```python
from build123d import *

# Parameters (mm, degrees)
SKETCH_2_OUTSIDE_W   = 46.494
SKETCH_2_OUTSIDE_H   = 46.494
SKETCH_2_OUTSIDE_W_2 = 10
SKETCH_2_OUTSIDE_H_2 = 5
CUT_EXTRUDE_1_DEPTH  = 10
SKETCH_3_OUTSIDE_W   = 46.494
SKETCH_3_OUTSIDE_H   = 46.494
SKETCH_3_OUTSIDE_W_2 = 5
SKETCH_3_OUTSIDE_H_2 = 20
CUT_EXTRUDE_2_DEPTH  = 8.5
CUT_EXTRUDE_3_DEPTH  = 131.817621137


with BuildPart() as part:
    # Эскиз1 → Повернуть2 (revolve)
    with BuildSketch(Plane.XY, mode=Mode.PRIVATE) as revolve_2_sk:
        with BuildLine():
            Line((-3.5, 8.570714214), (-3.5, 23.570714214))
            Line((-3.5, 23.570714214), (-9, 23.570714214))
            Line((-9, 23.570714214), (-9, 25.570714214))
            Line((-9, 25.570714214), (-1.5, 25.570714214))
            Line((-1.5, 25.570714214), (-1.5, 71.070714214))
            Line((-1.5, 71.070714214), (-6, 71.070714214))
            Line((-6, 71.070714214), (-6, 105.570714214))
            Line((-6, 105.570714214), (-9, 105.570714214))
            Line((-9, 105.570714214), (-9, 108.570714214))
            Line((-9, 108.570714214), (-8, 108.570714214))
            Line((-8, 108.570714214), (-8, 123.570714214))
            Line((-8, 123.570714214), (-4.791361199, 123.570714214))
            ThreePointArc((-4.791361199, 123.570714214), (-4.009141362, 127.987772671), (0, 130))
            Line((0, 130), (0, 125))
            Line((0, 125), (0, 0))
            ThreePointArc((0, 0), (-4.628907596, 3.109705191), (-3.5, 8.570714214))
        make_face()
    revolve(revolve_2_sk.sketch.rotate(Axis((0, 125, 0), (0, -1, 0)), 270), axis=Axis((0, 125, 0), (0, -1, 0)))

    # Эскиз2 outside → Вырез-Вытянуть1 (cut)
    with BuildSketch(Plane(origin=(0, 123.570714214, 0), x_dir=(1, 0, 0), z_dir=(0, 1, 0))):
        Rectangle(SKETCH_2_OUTSIDE_W, SKETCH_2_OUTSIDE_H)
        Rectangle(SKETCH_2_OUTSIDE_W_2, SKETCH_2_OUTSIDE_H_2, mode=Mode.SUBTRACT)
    extrude(amount=CUT_EXTRUDE_1_DEPTH, mode=Mode.SUBTRACT)

    # Эскиз3 outside → Вырез-Вытянуть2 (cut)
    with BuildSketch(Plane(origin=(0, 0, 0), x_dir=(1, 0, 0), z_dir=(0, 1, 0))):
        Rectangle(SKETCH_3_OUTSIDE_W, SKETCH_3_OUTSIDE_H)
        Rectangle(SKETCH_3_OUTSIDE_W_2, SKETCH_3_OUTSIDE_H_2, mode=Mode.SUBTRACT)
    extrude(amount=CUT_EXTRUDE_2_DEPTH, mode=Mode.SUBTRACT)

    # Эскиз4 → Вырез-Вытянуть3 (cut, through all)
    with BuildSketch(Plane(origin=(2.5, 0, 0), x_dir=(0, 0, -1), z_dir=(1, 0, 0))):
        with BuildLine():
            Line((-1.198957881, 7.334936491), (1.198957881, 7.334936491))
            ThreePointArc((1.198957881, 7.334936491), (3, 4.584936491), (1.198957881, 1.834936491))
            Line((1.198957881, 1.834936491), (-1.198957881, 1.834936491))
            ThreePointArc((-1.198957881, 1.834936491), (-3, 4.584936491), (-1.198957881, 7.334936491))
        make_face()
    extrude(amount=-CUT_EXTRUDE_3_DEPTH, mode=Mode.SUBTRACT)


solid = part.part
```
Input: part model. Units: mm. Frame: model coordinates. A direction names the side the tool comes from. Give positions to 0.01 mm unless a question says otherwise; leave off trailing zeros. Loops run counter-clockwise (first coordinate to the right, second up) from the corner with the lowest first, then second, coordinate; pieces in that order, holes last. Notation, with made-up numbers: (89.5, 79.5) -> (106.5, 79.5) arc R26 ccw to (106.5, 118.5) -> close; hole circle Ø3 at (57, 17.25). An arc over 180 degrees is marked (long way). Use a Markdown table: item, result.
Q1. Pull-direction query (Y, two-part tool) for faces 1 (the flat face through (0, 126, -2.5)), 2 (the flat face through (1.2, 71.071, -1.2)); classes: pulls with the +Y half, pulls with the -Y half, needs draft (parallel to the pull), parting line crosses it, or undercut.
Entries:
| item | result |
|---|---|
| face 1 | needs draft |
| face 2 | undercut |
Q2. Access query for faces 3 (the cylindrical face through (-0.45, 48.64, 1.43)), 4 (the flat face through (0, 126, 2.5)), 5 (the cylindrical face through (7.81, 116.18, -1.73)), 6 (the cylindrical face through (0, 4.6, -3)), 7 (the flat face through (2.5, 7.1, 2)). Directions: +Z, -Z, +X, -X, +Y, -Y. A direction counts if a zero-diameter tool reaches every point of the face in a straight line with its end or side. Return the directions, or none.
Entries:
| item | result |
|---|---|
| face 3 | none |
| face 4 | +Z, +X, -X, +Y |
| face 5 | +Y |
| face 6 | +X, -X |
| face 7 | +Z, -Z, +X, -Y |
Q3. Section query B-B, the plane y = 72.5. Return the cut outline in (x, z), plus the area to 3 significant figures.
Entries:
| item | result |
|---|---|
| outline | circle Ø12 at (0, 0) |
| area | 113 mm² |
Q4. Ray query, probe 1 along Y at (x, z) = (-4.75, -3.25); probe 2 along Y at (x, z) = (7.25, 5.25); probe 3 along Y at (x, z) = (1.25, 2.25). Return the intervals inside material, ascending. Write a range as from..to.
Entries:
| item | result |
|---|---|
| probe 1 | y = 23.57..25.57, 71.07..123.57 |
| probe 2 | y = 23.57..25.57, 105.57..108.57 |
| probe 3 | y = 0.71..2.6, 6.57..25.57, 71.07..129.29 |
Q5. First-contact query: P1, Ø8.5, axis at y = 4, z = -1.5, coming from the -X side; P2, Ø0.7, axis at x = -0.5, z = -0.5, coming from the -Y side; P3, Ø6.5, axis at x = -2, y = 126, coming from the +Z side; P4, Ø1.2, axis at x = -0.5, z = 0, coming from the +Y side. Flat tips, straight axial feed; report the tip coordinate or a pass-through.
Entries:
| item | result |
|---|---|
| P1 | stops at x = -2.5 |
| P2 | stops at y = 0.01 |
| P3 | stops at z = 8 |
| P4 | stops at y = 130 |
